Can you work these out from the model? Positions are in its coordinate system, mm. A direction names the side the tool comes from. Round coordinates to 2 decimals unless told otherwise and drop trailing zeros. Order: outer loops, then holes, each group sorted by start corner. A loop starts at its lowest first (then second) coordinate and runs counter-clockwise, first axis right, second up. Notation, with made-up numbers: M -7.75,-39 L 25.25,-39 A29 cw 25.25,-3 Z; hole C 49,-39.75 d6. An arc over 180 degrees is marked long. Answer as CSV lines item,"result". Start each with the question number.
Autodesk Inventor part; units mm, degrees
ref_plane "YZ Plane" through (0, 0, 0) normal (1, 0, 0) x (0, 1, 0)
ref_plane "XZ Plane" through (0, 0, 0) normal (0, 1, 0) x (-1, 0, 0)
ref_plane "XY Plane" through (0, 0, 0) normal (0, 0, 1) x (1, 0, 0)
sketch "Skizze1" plane through (0, 0, 0) normal (0, 0, 1) x (1, 0, 0)
  line L0 (0, 0) -> (20.8, 0)
  line L1 (20.8, 0) -> (20.8, 20.1)
  line L2 (20.8, 20.1) -> (0, 20.1)
  line L3 (0, 20.1) -> (0, 0)
  arc A0 (2.8586, 27.1) -> (0, 20.1) centre (10, 20.1) ccw
  line L4 (2.8586, 27.1) -> (17.9414, 27.1)
  arc A1 (20.8, 20.1) -> (17.9414, 27.1) centre (10.8, 20.1) ccw
  circle A2 centre (4.95, 24.4) radius 1.95
  circle A3 centre (15.85, 24.4) radius 1.95
  line L5 (4.95, 26.35) -> (15.85, 26.35) construction
  point P0 (10.4, 27.1)
  dimension "d4" = 3.9
  dimension "d0" = 27.1
  dimension "d1" = 20.8
  dimension "d2" = 7
  dimension "d3" = 10
  dimension "d5" = 10.9
  dimension "d6" = 5.45
  dimension "d7" = 26.35
extrude "Extrusion1" add sketch "Skizze1" along normal blind 10.2 contours L3 L2 L1 L0 | A0 L4 A1 L2 | A2 | A3
extrude "Extrusion2" add sketch "Skizze1" against normal blind 3 contours A2 | A3
fillet "Rundung1" radius 7 1 edges at (10.4, 27.1, 10.2)
chamfer "Fase1" distance 0.5 angle 45 2 edges at (13.9, 24.4, -3) (3, 24.4, -3)
sketch "Skizze2" plane through (0, 0, 0) normal (0, -1, 0) x (1, 0, 0)
  line L0 (0.5, 0.65) -> (0.5, 9.55)
  line L1 (0.5, 9.55) -> (17.35, 9.55)
  line L2 (17.35, 9.55) -> (20.3, 6.6)
  line L3 (20.3, 6.6) -> (20.3, 3.6)
  line L4 (20.3, 3.6) -> (17.35, 0.65)
  line L5 (0.5, 0.65) -> (17.35, 0.65)
  line L6 (0, 0) -> (0, 10.2)
  circle A0 centre (4.95, 5.1) radius 2.85
  circle A1 centre (4.95, 5.1) radius 2.25
  circle A2 centre (15.85, 5.1) radius 2.85
  circle A3 centre (15.85, 5.1) radius 2.25
  line L7 (0, 10.2) -> (20.8, 10.2)
  point P0 (0.5, 5.1)
  point P1 (0, 5.1)
  point P2 (20.3, 5.1)
  point P3 (10.4, 10.2)
  dimension "d16" = 19.8
  dimension "d17" = 8.9
  dimension "d18" = 0.5
  dimension "d19" = 3
  dimension "d20" = 45
  dimension "d21" = 5.7
  dimension "d22" = 4.5
  dimension "d23" = 10.9
  dimension "d24" = 5.45
extrude "Extrusion3" cut sketch "Skizze2" against normal blind 11 contours L0 L1 L2 L3 L4 L5 | A0 | A2
chamfer "Fase2" distance 0.5 angle 45 2 edges at (2.7, 0, 5.1) (13.6, 0, 5.1)
properties part number "XT90PW" material "PC/ABS-Kunststoff"
(1) If I drill on line 1 along Z through (x, y) = (11, 3.5); line 2 along Z through (x, y) = (17, 1.5); line 3 along Z through (x, y) = (14, 18.25), over which ranges is the centre line in solid material (lowest first)?
(2) For faces 4 (the cylindrical face through (17.996, 5.676, 5.776)), 5 (the flat face through (11.9, 0, 0.5)), 6 (the cylindrical face through (16.898, 26.044, -1.232)), which set-ups out of +Z, -Z, +X, -X, +Y, -Y let a thin tool reach every point of the face, with its end or its side?
(3) I want a section at D-D on z = 5.1. Write out the boundary of the cut face in (x, y).
(4) I want a section at A-A on y = 5.25. Write out the boundary of the cut face in (x, z).
(5) If we mould it in two halves opening along Z, with no side actions, what happens to faces 1 (the cylindrical face through (10.5, 25.1, 8.1)), 2 (the flat face through (10, 14, 0)), 3 (the flat face through (20.3, 5, 5))? For each: +Z half, -Z half, draft (parallel to the pull), parting line (faces both ways), or undercut.
(6) I want a section at B-B on x = 12.75. Write out the boundary of the cut face in (y, z), and give its area (3 significant figures).
(7) I want a section at C-C on z = -1.25. Write out the boundary of the cut face in (x, y).
(8) I'm going to push flat-ended pins straight in: P1, Ø1, axis at x = 17.5, y = 7.5, coming from the -Z side; P2, Ø4.5, axis at x = 10, z = 4.5, coming from the -Y side. Where does each tip first touch, or does it pass through?
From the geometry:
1,line 1,"0 to 0.65, 9.55 to 10.2"
1,line 2,"0 to 0.65, 3.17 to 7.03, 9.55 to 10.2"
1,line 3,"0 to 10.2"
2,face 4,"-Y"
2,face 5,"+Z, -Z, +X, -X, -Y"
2,face 6,"-Z"
3,outline,"M 0,0 L 0.5,0 L 0.5,11 L 2.7,11 L 2.7,0.5 L 3.2,0 L 6.7,0 L 7.2,0.5 L 7.2,11 L 13.6,11 L 13.6,0.5 L 14.1,0 L 17.6,0 L 18.1,0.5 L 18.1,11 L 20.3,11 L 20.3,0 L 20.8,0 L 20.8,20.1 A10 ccw 18.19,26.84 L 2.61,26.84 A10 ccw 0,20.1 Z"
4,outline,"M 0,0 L 20.8,0 L 20.8,10.2 L 0,10.2 Z; C 4.95,5.1 d4.5; C 15.85,5.1 d4.5; hole M 0.5,0.65 L 17.35,0.65 L 20.3,3.6 L 20.3,6.6 L 17.35,9.55 L 0.5,9.55 Z"
5,face 1,"+Z half"
5,face 2,"-Z half"
5,face 3,"undercut"
6,outline,"M 0,0 L 27.1,0 L 27.1,3.2 A7 ccw 20.1,10.2 L 0,10.2 L 0,9.55 L 11,9.55 L 11,0.65 L 0,0.65 Z"
6,area,"168 mm²"
7,outline,"C 4.95,24.4 d3.9; C 15.85,24.4 d3.9"
8,P1,"z = 0"
8,P2,"y = 11"
